Part model, mm, in its own coordinate system. Face numbers are marked on the shaded views. A direction names the side the tool comes from. Round coordinates to 2 decimals unless told otherwise and drop trailing zeros. Order: outer loops, then holes, each group sorted by start corner. A loop starts at its lowest first (then second) coordinate and runs counter-clockwise, first axis right, second up. Notation, with made-up numbers: M 39,34 L 64,34 A28 ccw 64,71 Z; hole C 22.25,34.25 d3. An arc over 180 degrees is marked long. One line per question, with ' | ' between items.
from build123d import *

# Parameters (mm, degrees)
SKETCH_1_W             = 30.8
SKETCH_1_H             = 12.6
EXTRUDE_1_DEPTH        = 1.2
EXTRUDE_2_DEPTH        = 6.1
EXTRUDE_3_DEPTH        = 10
SKETCH_5_W             = 0.3556
SKETCH_5_H             = 6.1
SKETCH_6_W             = 0.3556
SKETCH_6_H             = 6.1
PATTERN_LINEAR_1_COUNT = 5
PATTERN_LINEAR_1_PITCH = 2.54
PATTERN_LINEAR_2_COUNT = 4
PATTERN_LINEAR_2_PITCH = 2.54
HOLE_WIZARD_3_2_D      = 3.048
FILLET_1_R             = 1


with BuildPart() as part:
    # ｽｹｯﾁ1 → ﾎﾞｽ - 押し出し1 (new body)
    with BuildSketch(Plane.XY):
        Rectangle(SKETCH_1_W, SKETCH_1_H)
    extrude(amount=EXTRUDE_1_DEPTH)

    # ｽｹｯﾁ2 → ﾎﾞｽ - 押し出し2 (add)
    with BuildSketch(Plane.XY.offset(1.2)):
        Polygon((-6.751123011, -3.91), (6.751123011, -3.91), (8.13, 3.91), (-8.13, 3.91), align=None)
    extrude(amount=EXTRUDE_2_DEPTH)

    # ｽｹｯﾁ3 → ﾎﾞｽ - 押し出し3 (add)
    with BuildSketch(Plane(origin=(0, 0, 0), x_dir=(-1, 0, 0), z_dir=(0, 0, -1))):
        Polygon((-7.763301306, -5.35), (7.763301306, -5.35), (9.65, 5.35), (-9.65, 5.35), align=None)
    extrude(amount=EXTRUDE_3_DEPTH)

    # ｽｹｯﾁ5 → #0000 すきま穴1 (revolve, cut)
    with BuildSketch(Plane(origin=(-4.225439316, 1.008007938, 1.2), x_dir=(0, 1, 0), z_dir=(1, 0, 0))):
        with Locations((0.1778, 3.05)):
            Rectangle(SKETCH_5_W, SKETCH_5_H)
    hole_wizard_0000_1 = revolve(axis=Axis((-4.225439316, 1.008007938, -5.15), (0, 0, 1)), mode=Mode.SUBTRACT)

    # ｽｹｯﾁ6 → #0000 すきま穴2 (revolve, cut)
    with BuildSketch(Plane(origin=(-3.168321124, -1.202810505, 1.2), x_dir=(0, 1, 0), z_dir=(1, 0, 0))):
        with Locations((0.1778, 3.05)):
            Rectangle(SKETCH_6_W, SKETCH_6_H)
    hole_wizard_0000_2 = revolve(axis=Axis((-3.168321124, -1.202810505, -5.15), (0, 0, 1)), mode=Mode.SUBTRACT)

    # 直線ﾊﾟﾀｰﾝ1: #0000 すきま穴1 ×5
    with Locations(*[(i * PATTERN_LINEAR_1_PITCH, 0, 0) for i in range(1, PATTERN_LINEAR_1_COUNT)]):
        add(hole_wizard_0000_1, mode=Mode.SUBTRACT)

    # 直線ﾊﾟﾀｰﾝ2: #0000 すきま穴2 ×4
    with Locations(*[(i * PATTERN_LINEAR_2_PITCH, 0, 0) for i in range(1, PATTERN_LINEAR_2_COUNT)]):
        add(hole_wizard_0000_2, mode=Mode.SUBTRACT)

    # #3 すきま穴2 (through all)
    with Locations(Plane(origin=(-12.495, 0, 1.2), x_dir=(1, 0, 0), z_dir=(0, 0, 1))):
        with Locations((0, 0), (24.99, 0)):
            Hole(HOLE_WIZARD_3_2_D / 2)

    # ﾌｨﾚｯﾄ1
    fillet_1_edges = [part.edges().sort_by_distance(p)[0] for p in [
        (6.751123011, -3.91, 4.25),
        (8.13, 3.91, 4.25),
        (-8.13, 3.91, 4.25),
        (-6.751123011, -3.91, 4.25),
        (-7.763301306, -5.35, -5),
        (-9.65, 5.35, -5),
        (9.65, 5.35, -5),
        (7.763301306, -5.35, -5),
    ]]
    fillet(fillet_1_edges, radius=FILLET_1_R)


solid = part.part
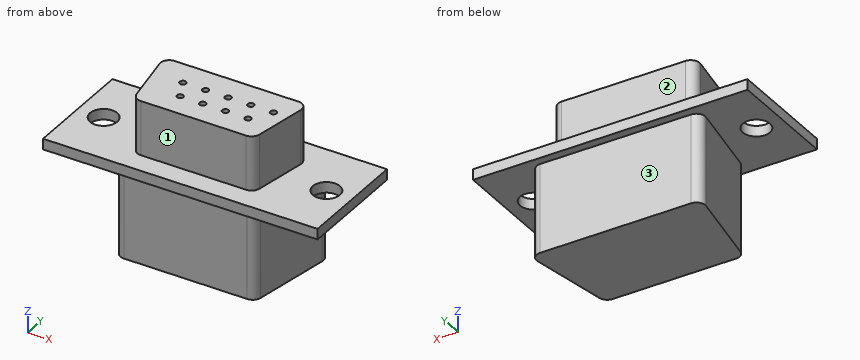
1) Drop flat-ended pins along their axis: pin 1 (3 mm diameter, centred on x = -0.5, z = 5, fed in from +Y); pin 2 (0.6 mm diameter, centred on x = 4.5, y = -1.5, fed in from +Z); pin 3 (4 mm diameter, centred on x = 12.495, y = 0, fed in from +Z); pin 4 (8 mm diameter, centred on x = 12, z = -4.5, fed in from +Y). Give the stop position or say it passes through.
The answers:
pin 1: stops at y = 3.91 | pin 2: stops at z = 7.3 | pin 3: stops at z = 1.2 | pin 4: stops at y = 5.35
2) Saw through at B-B (y = 0). List the corners of the cut face in (x, z).
The answers:
outline: M -15.4,0 L -14.02,0 L -14.02,1.2 L -15.4,1.2 Z; M -10.97,0 L -8.71,0 L -8.71,-10 L 8.71,-10 L 8.71,0 L 10.97,0 L 10.97,1.2 L 7.44,1.2 L 7.44,7.3 L -7.44,7.3 L -7.44,1.2 L -10.97,1.2 Z; M 14.02,0 L 15.4,0 L 15.4,1.2 L 14.02,1.2 Z
3) Saw through at C-C (z = 5.25). Give the number of separate pieces and of enclosed holes in the cut face, plus the area to 3 significant figures.
The answers:
separate pieces: 1 | enclosed holes: 9 | area: 112 mm²
4) Probe line 1 (Y direction, x = 3, z = -4.5); line 2 (X direction, y = 0.25, z = 1); line 3 (Y direction, x = 2, z = 5.5). List the from-to ranges inside material, lowest first. Write a range as [from, to].
The answers:
line 1: y = [-5.35, 5.35] | line 2: x = [-15.4, -14], [-10.99, 10.99], [14, 15.4] | line 3: y = [-3.91, -1.55], [-0.86, 3.91]
5) Saw through at D-D (x = -10.5). List the corners of the cut face in (y, z), plus the area to 3 significant figures.
The answers:
outline: M -6.3,0 L 6.3,0 L 6.3,1.2 L -6.3,1.2 Z | area: 15.1 mm²
6) Which spindle directions (+Z, -Z, +X, -X, +Y, -Y) get a long thin tool onto all of the face, cutting with end or side? Do the marked faces 1, 2 and 3. Say none if no direction does.
The answers:
face 1: +Z, +X, -X, -Y | face 2: +Z, +X, -X, +Y | face 3: -Z, +X, -X, +Y
7) Saw through at A-A (z = -1.25). List the corners of the cut face in (x, y).
The answers:
outline: M -9.44,4.18 L -7.91,-4.52 A1 ccw -6.92,-5.35 L 6.92,-5.35 A1 ccw 7.91,-4.52 L 9.44,4.18 A1 ccw 8.46,5.35 L -8.46,5.35 A1 ccw Z
